Design review of the part built by this model. Coordinates are the model's own, in mm. Give positions to 0.01 mm unless a question says otherwise; leave off trailing zeros. Loops run counter-clockwise (first coordinate to the right, second up) from the corner with the lowest first, then second, coordinate; pieces in that order, holes last. Notation, with made-up numbers: (-14, -37) -> (11, -37) arc R11 ccw to (11, -25) -> close; hole circle Ø10 at (-40, 38). An arc over 180 degrees is marked (long way). Answer in a Markdown table with one row per item. Add a question column.
(1) Consider section A-A on x = 0. Write out the cut boundary in (y, z), then the cut area to 3 significant figures.
(2) Consider section B-B on y = 28.5. Write out the cut boundary in (x, z).
(3) For pin 1 (1.5 mm diameter, centred on y = -8.5, z = 1.5, fed in from +X); pin 2 (8 mm diameter, centred on x = -22.5, y = 0.5, fed in from -Z); pin 3 (1.5 mm diameter, centred on x = -21, z = 5, fed in from -Y), all flat-tipped, find the tip position at first contact; note any pin that passes through.
(4) Consider section C-C on z = 5. Write out the cut boundary in (x, y), then the cut area to 3 significant figures.
(5) For line 1 (Y direction, x = 0, z = 2.75); line 2 (X direction, y = -49, z = 0.75); line 3 (X direction, y = 34.5, z = 0.5), list the stretches that pass through material, from the lowest coordinate up.
(6) Consider section D-D on x = -19. Write out the cut boundary in (y, z), then the cut area to 3 significant figures.
from build123d import *

# Parameters (mm, degrees)
F0_R     = 11.267098278
F0_R_2   = 12.3387041608
F1_DEPTH = 6.35


with BuildPart() as f1:
    # F0 (on Top) → F1 (new body)
    with BuildSketch(Plane.XY):
        with BuildLine():
            ThreePointArc((8.7123179944, 15.0903645105), (4.9401614153, 25.5916315175), (7.8734188263, 36.3574001836))
            ThreePointArc((7.8734188263, 36.3574001836), (-0.9009997096, 64.4580259045), (-6.2804322517, 35.5150251603))
            ThreePointArc((-6.2804322517, 35.5150251603), (-5.1328327, 25.0212030543), (-8.7124800213, 15.0902709642))
            ThreePointArc((-8.7124800213, 15.0902709642), (-19.6929223108, 17.0741210432), (-27.5497227614, 24.99728081))
            ThreePointArc((-27.5497227614, 24.99728081), (-56.2727877659, 31.4487243149), (-33.8971301307, 12.3184987035))
            ThreePointArc((-33.8971301307, 12.3184987035), (-24.2354138283, 8.0654380156), (-17.4247980157, -9.35463e-05))
            ThreePointArc((-17.4247980157, -9.35463e-05), (-24.6330837261, -8.5175104743), (-35.4231415877, -11.3601193736))
            ThreePointArc((-35.4231415877, -11.3601193736), (-55.3717880563, -33.0093015896), (-27.6166978791, -23.1965264569))
            ThreePointArc((-27.6166978791, -23.1965264569), (-19.1025811283, -16.9557650387), (-8.7123179944, -15.0903645105))
            ThreePointArc((-8.7123179944, -15.0903645105), (-4.9401614153, -25.5916315175), (-7.8734188263, -36.3574001836))
            ThreePointArc((-7.8734188263, -36.3574001836), (0.9009997096, -64.4580259045), (6.2804322517, -35.5150251603))
            ThreePointArc((6.2804322517, -35.5150251603), (5.1328327, -25.0212030543), (8.7124800213, -15.0902709642))
            ThreePointArc((8.7124800213, -15.0902709642), (19.6929223108, -17.0741210432), (27.5497227614, -24.99728081))
            ThreePointArc((27.5497227614, -24.99728081), (56.2727877659, -31.4487243149), (33.8971301307, -12.3184987035))
            ThreePointArc((33.8971301307, -12.3184987035), (24.2354138283, -8.0654380156), (17.4247980157, 9.35463e-05))
            ThreePointArc((17.4247980157, 9.35463e-05), (24.6330837261, 8.5175104743), (35.4231415877, 11.3601193736))
            ThreePointArc((35.4231415877, 11.3601193736), (55.3717880563, 33.0093015896), (27.6166978791, 23.1965264569))
            ThreePointArc((27.6166978791, 23.1965264569), (19.1025811283, 16.9557650387), (8.7123179944, 15.0903645105))
        make_face()
        with Locations((-42.7116318899, -24.6595721692)):
            Circle(F0_R, mode=Mode.SUBTRACT)
        with BuildLine():
            ThreePointArc((-8.3770879832, -15.1094843982), (-8.5446687054, -15.0993233615), (-8.7123179944, -15.0903645105))
            ThreePointArc((-8.7123179944, -15.0903645105), (-8.8358376955, -14.9298053557), (-8.9611030536, -14.7706043858))
            ThreePointArc((-8.9611030536, -14.7706043858), (-8.6707512375, -14.9428978058), (-8.3770879832, -15.1094843982))
        make_face(mode=Mode.SUBTRACT)
        with Locations((0, -49.3191443384)):
            Circle(F0_R, mode=Mode.SUBTRACT)
        with BuildLine():
            ThreePointArc((8.8966533354, -14.8095132023), (8.8040632583, -14.9495618465), (8.7124800213, -15.0902709642))
            ThreePointArc((8.7124800213, -15.0902709642), (8.5116718638, -15.1169625859), (8.3111671005, -15.1458450832))
            ThreePointArc((8.3111671005, -15.1458450832), (8.6055534873, -14.9805397445), (8.8966533354, -14.8095132023))
        make_face(mode=Mode.SUBTRACT)
        with BuildLine():
            ThreePointArc((17.2737413186, 0.2999711959), (17.3487319637, 0.149761515), (17.4247980157, 9.35463e-05))
            ThreePointArc((17.4247980157, 9.35463e-05), (17.3475095593, -0.1871572302), (17.2722701541, -0.3752406974))
            ThreePointArc((17.2722701541, -0.3752406974), (17.2763047248, -0.0376419387), (17.2737413186, 0.2999711959))
        make_face(mode=Mode.SUBTRACT)
        with Locations((42.7116318899, -24.6595721692)):
            Circle(F0_R, mode=Mode.SUBTRACT)
        with Locations((-42.7116318899, 24.6595721692)):
            Circle(F0_R, mode=Mode.SUBTRACT)
        with BuildLine():
            ThreePointArc((-17.2737413186, -0.2999711959), (-17.3487319637, -0.149761515), (-17.4247980157, -9.35463e-05))
            ThreePointArc((-17.4247980157, -9.35463e-05), (-17.3475095593, 0.1871572302), (-17.2722701541, 0.3752406974))
            ThreePointArc((-17.2722701541, 0.3752406974), (-17.2763047248, 0.0376419387), (-17.2737413186, -0.2999711959))
        make_face(mode=Mode.SUBTRACT)
        Circle(F0_R_2, mode=Mode.SUBTRACT)
        with Locations((42.7116318899, 24.6595721692)):
            Circle(F0_R, mode=Mode.SUBTRACT)
        with Locations((0, 49.3191443384)):
            Circle(F0_R, mode=Mode.SUBTRACT)
        with BuildLine():
            ThreePointArc((-17.2722701541, 0.3752406974), (-17.3475095593, 0.1871572302), (-17.4247980157, -9.35463e-05))
            ThreePointArc((-17.4247980157, -9.35463e-05), (-17.3487319637, -0.149761515), (-17.2737413186, -0.2999711959))
            ThreePointArc((-17.2737413186, -0.2999711959), (-17.2763047248, 0.0376419387), (-17.2722701541, 0.3752406974))
        make_face()
        with BuildLine():
            ThreePointArc((-8.9611030536, -14.7706043858), (-8.8358376955, -14.9298053557), (-8.7123179944, -15.0903645105))
            ThreePointArc((-8.7123179944, -15.0903645105), (-8.5446687054, -15.0993233615), (-8.3770879832, -15.1094843982))
            ThreePointArc((-8.3770879832, -15.1094843982), (-8.6707512375, -14.9428978058), (-8.9611030536, -14.7706043858))
        make_face()
        with BuildLine():
            ThreePointArc((8.3111671005, -15.1458450832), (8.5116718638, -15.1169625859), (8.7124800213, -15.0902709642))
            ThreePointArc((8.7124800213, -15.0902709642), (8.8040632583, -14.9495618465), (8.8966533354, -14.8095132023))
            ThreePointArc((8.8966533354, -14.8095132023), (8.6055534873, -14.9805397445), (8.3111671005, -15.1458450832))
        make_face()
        with BuildLine():
            ThreePointArc((17.2722701541, -0.3752406974), (17.3475095593, -0.1871572302), (17.4247980157, 9.35463e-05))
            ThreePointArc((17.4247980157, 9.35463e-05), (17.3487319637, 0.149761515), (17.2737413186, 0.2999711959))
            ThreePointArc((17.2737413186, 0.2999711959), (17.2763047248, -0.0376419387), (17.2722701541, -0.3752406974))
        make_face()
    extrude(amount=F1_DEPTH)


solid = f1.part
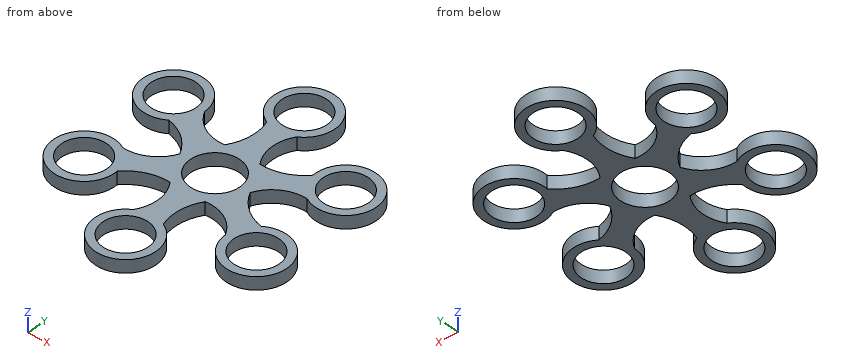
Values follow:
| question | item | result |
|---|---|---|
| 1 | outline | (-64.48, 0) -> (-60.59, 0) -> (-60.59, 6.35) -> (-64.48, 6.35) -> close; (-38.05, 0) -> (-12.34, 0) -> (-12.34, 6.35) -> (-38.05, 6.35) -> close; (12.34, 0) -> (38.05, 0) -> (38.05, 6.35) -> (12.34, 6.35) -> close; (60.59, 0) -> (64.48, 0) -> (64.48, 6.35) -> (60.59, 6.35) -> close |
| 1 | area | 376 mm2 |
| 2 | outline | (-57.38, 0) -> (-53.3, 0) -> (-53.3, 6.35) -> (-57.38, 6.35) -> close; (-32.12, 0) -> (-28.04, 0) -> (-28.04, 6.35) -> (-32.12, 6.35) -> close; (-4.98, 0) -> (5.05, 0) -> (5.05, 6.35) -> (-4.98, 6.35) -> close; (28.04, 0) -> (32.12, 0) -> (32.12, 6.35) -> (28.04, 6.35) -> close; (53.3, 0) -> (57.38, 0) -> (57.38, 6.35) -> (53.3, 6.35) -> close |
| 3 | pin 1 | x = 25.98 |
| 3 | pin 2 | through |
| 3 | pin 3 | y = -18.3 |
| 4 | outline | (-35.42, -11.36) arc R15.17 ccw (long way) to (-27.62, -23.2) arc R23.41 cw to (-8.71, -15.09) arc R18.55 cw to (-7.87, -36.36) arc R15.17 ccw (long way) to (6.28, -35.52) arc R23.41 cw to (8.71, -15.09) arc R18.55 cw to (27.55, -25) arc R15.17 ccw (long way) to (33.9, -12.32) arc R23.41 cw to (17.42, 0) arc R18.55 cw to (35.42, 11.36) arc R15.17 ccw (long way) to (27.62, 23.2) arc R23.41 cw to (8.71, 15.09) arc R18.55 cw to (7.87, 36.36) arc R15.17 ccw (long way) to (-6.28, 35.52) arc R23.41 cw to (-8.71, 15.09) arc R18.55 cw to (-27.55, 25) arc R15.17 ccw (long way) to (-33.9, 12.32) arc R23.41 cw to (-17.42, 0) arc R18.55 cw to start; hole circle Ø22.53 at (-42.71, -24.66); hole circle Ø22.53 at (-42.71, 24.66); hole circle Ø24.68 at (0, 0); hole circle Ø22.53 at (0, -49.32); hole circle Ø22.53 at (0, 49.32); hole circle Ø22.53 at (42.71, -24.66); hole circle Ø22.53 at (42.71, 24.66) |
| 4 | area | 3,640 mm2 |
| 5 | line 1 | -64.48 to -60.59, -38.05 to -12.34, 12.34 to 38.05, 60.59 to 64.48 |
| 5 | line 2 | -15.16 to -11.26, 11.26 to 15.16 |
| 5 | line 3 | -54.25 to -48.2, -37.22 to -31.17, -5.95 to 6.82, 31.17 to 37.22, 48.2 to 54.25 |
| 6 | outline | (-16.91, 0) -> (-2.97, 0) -> (-2.97, 6.35) -> (-16.91, 6.35) -> close; (2.63, 0) -> (16.73, 0) -> (16.73, 6.35) -> (2.63, 6.35) -> close |
| 6 | area | 178 mm2 |
